For this review, use the dimensioned drawing (mm, ordinates from the lowest corner) and the shaded views. Coordinates: 2 decimals unless noted, no trailing zeros. Write each loop counter-clockwise with the first axis right and the second up, starting at its lowest first coordinate (ties: lowest second). Pieces come first, ordered by that corner, then holes. Notation, with made-up numbers: M 27.5,64.25 L 53.5,64.25 A11 cw 53.5,75.25 Z; hole C 24,5.5 d7. An arc over 180 degrees is marked long. One line per question, with ' | ' between items.
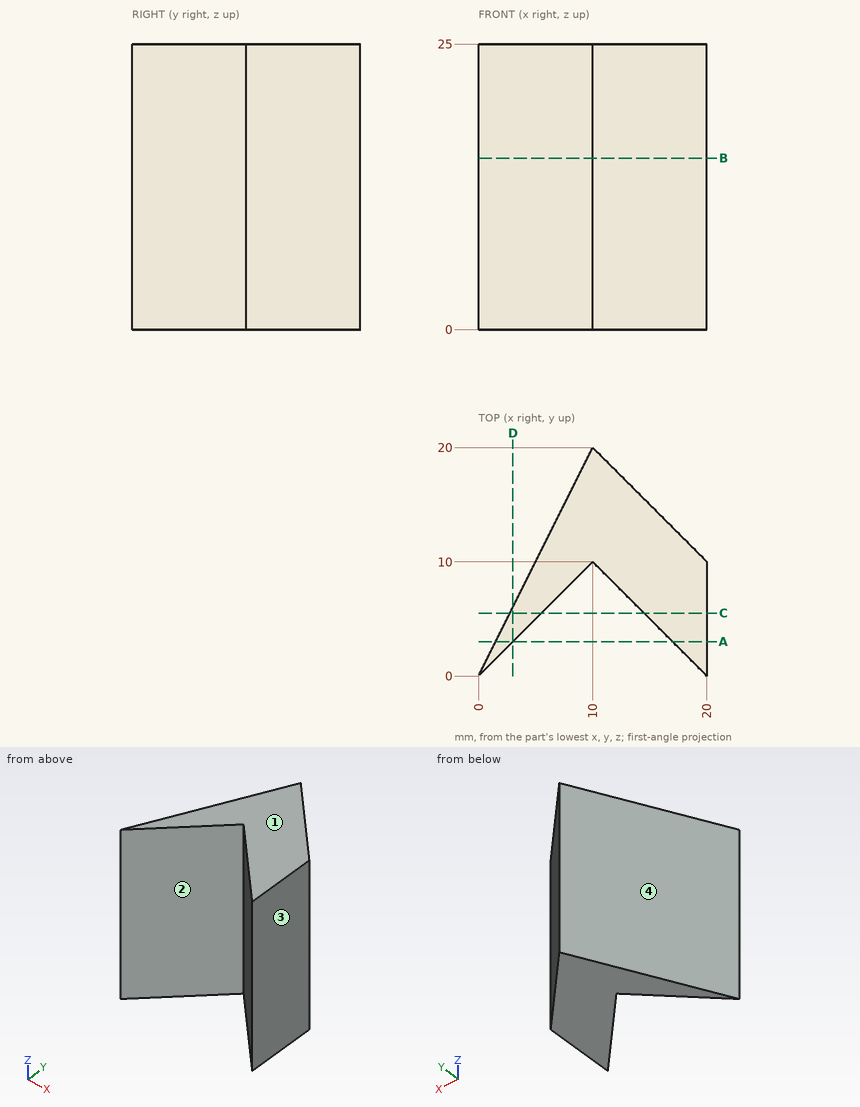
1. Take a section at A-A (y = 3). Write out the cut boundary in (x, z).
Answer sheet:
outline: M 1.5,0 L 3,0 L 3,25 L 1.5,25 Z; M 17,0 L 20,0 L 20,25 L 17,25 Z
2. To check wall thickness, follow line 1 along X through (y, z) = (9.5, 14); line 2 along X through (y, z) = (6.5, 11.5); line 3 along Y through (x, z) = (17, 8). State the ranges of each line that lie inside material, in increasing order. Write a range as [from, to].
Answer sheet:
line 1: [4.75, 9.5], [10.5, 20] | line 2: [3.25, 6.5], [13.5, 20] | line 3: [3, 13]
3. Take a section at D-D (x = 3). Write out the cut boundary in (y, z).
Answer sheet:
outline: M 3,0 L 6,0 L 6,25 L 3,25 Z
4. Draft analysis for pull direction X (two halves, no side actions). For the marked faces 1, 2, 3 and 4, state which applies: pulls with the +X half, pulls with the -X half, needs draft (parallel to the pull), parting line crosses it, or undercut.
Answer sheet:
face 1: needs draft | face 2: undercut | face 3: pulls with the +X half | face 4: pulls with the -X half
5. Take a section at C-C (y = 5.5). Write out the cut boundary in (x, z).
Answer sheet:
outline: M 2.75,0 L 5.5,0 L 5.5,25 L 2.75,25 Z; M 14.5,0 L 20,0 L 20,25 L 14.5,25 Z
6. Take a section at B-B (z = 15). Write out the cut boundary in (x, y), then the cut area to 3 significant figures.
Answer sheet:
outline: M 0,0 L 10,10 L 20,0 L 20,10 L 10,20 Z | area: 150 mm^2
7. Insertion check: pin 1 Ø1 at (y, z) = (12.5, 22) entering from -X; pin 2 Ø3 at (y, z) = (4, 18) entering from -X; pin 3 Ø2 at (y, z) = (5, 18.5) entering from -X. Each pin has a flat end and moves straight along its axis. Give the tip position at first contact, or say it passes through.
Answer sheet:
pin 1: x = 6 | pin 2: x = 1.25 | pin 3: x = 2
